For this review, use the dimensioned drawing (mm, ordinates from the lowest corner) and the shaded views. A direction names the side the tool comes from. Round coordinates to 2 decimals unless told otherwise and drop trailing zeros. Order: outer loops, then holes, each group sorted by start corner. A loop starts at its lowest first (then second) coordinate and runs counter-clockwise, first axis right, second up. Notation, with made-up numbers: (-29, 7) - (4, 7) arc R15 cw to (4, 20) - close; hole circle Ø4 at (24.5, -8). An arc over 180 degrees is marked (long way). Write item = value, one per line.
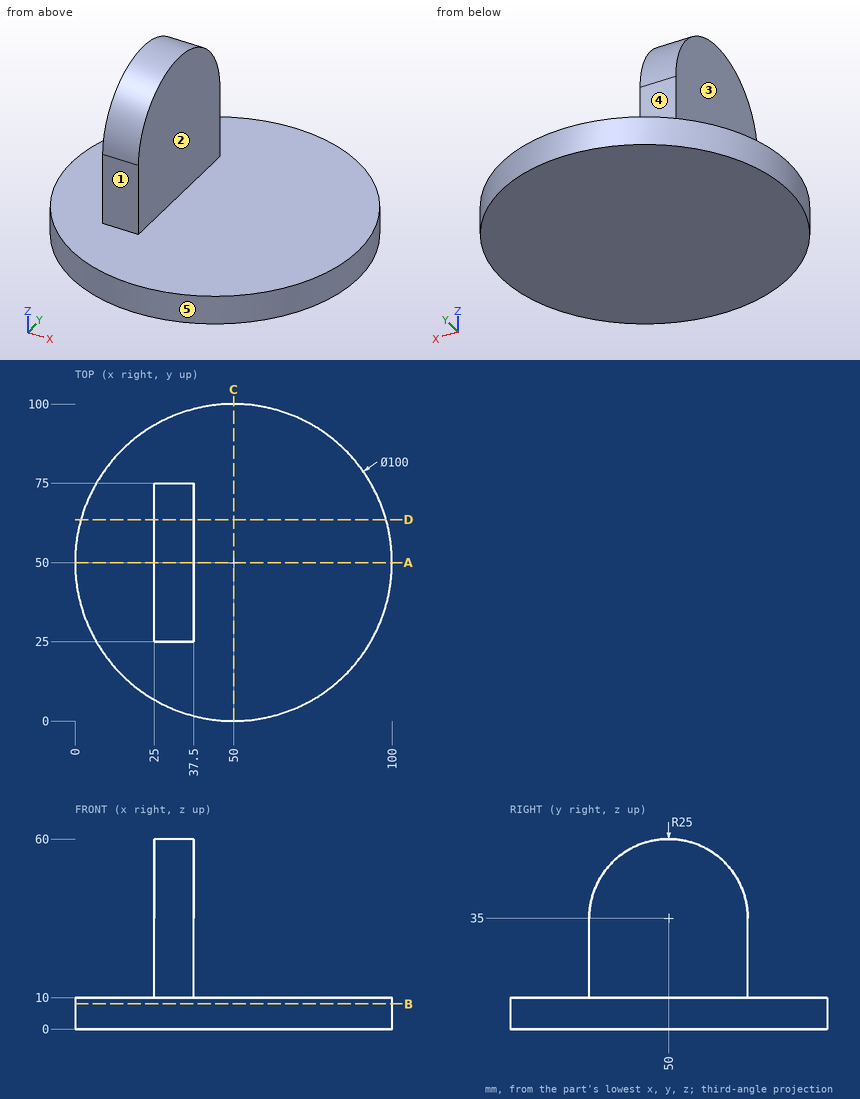
1) We need section B-B on z = 8. Write out the cut boundary in (x, y).
Findings:
outline = circle Ø100 at (50, 50)
2) Clearance check with flat-ended pins moving along their axes: pin 1 Ø10 at (x, z) = (33.5, 18) entering from +Y; pin 2 Ø12 at (y, z) = (27, 53.5) entering from +X; pin 3 Ø1 at (y, z) = (66.5, 50) entering from -X; pin 4 Ø12 at (x, y) = (87.5, 73.5) entering from -Z. State where each tip first meets the part, or that it passes through.
Findings:
pin_1 = 75
pin_2 = 37.5
pin_3 = 25
pin_4 = 0
3) To check wall thickness, follow L1, parallel to X at y = 63.5, z = 42; L2, parallel to Y at x = 30.5, z = 19.5; L3, parallel to Z at x = 13, y = 26. State the ranges of each line that lie inside material, in increasing order. Write a range as from..to.
Findings:
L1 = 25..37.5
L2 = 25..75
L3 = 0..10
4) We need section C-C on x = 50. Write out the cut boundary in (y, z).
Findings:
outline = (0, 0) - (100, 0) - (100, 10) - (0, 10) - close
5) We need section D-D on y = 63.5. Write out the cut boundary in (x, z).
Findings:
outline = (1.86, 0) - (98.14, 0) - (98.14, 10) - (37.5, 10) - (37.5, 56.04) - (25, 56.04) - (25, 10) - (1.86, 10) - close
6) For the marked faces 1, 2, 3, 4 and 5, list the 3-axis set-ups (+Z, -Z, +X, -X, +Y, -Y) from which the entire face can be reached by the end or side of a thin tool; tool diameter is ignored.
Findings:
face_1 = +Z, +X, -X, -Y
face_2 = +Z, +X, +Y, -Y
face_3 = +Z, -X, +Y, -Y
face_4 = +Z, +X, -X, +Y
face_5 = +Z, -Z
7) We need section A-A on y = 50. Write out the cut boundary in (x, z), and give its area (4 significant figures).
Findings:
outline = (0, 0) - (100, 0) - (100, 10) - (37.5, 10) - (37.5, 60) - (25, 60) - (25, 10) - (0, 10) - close
area = 1,625 mm^2
